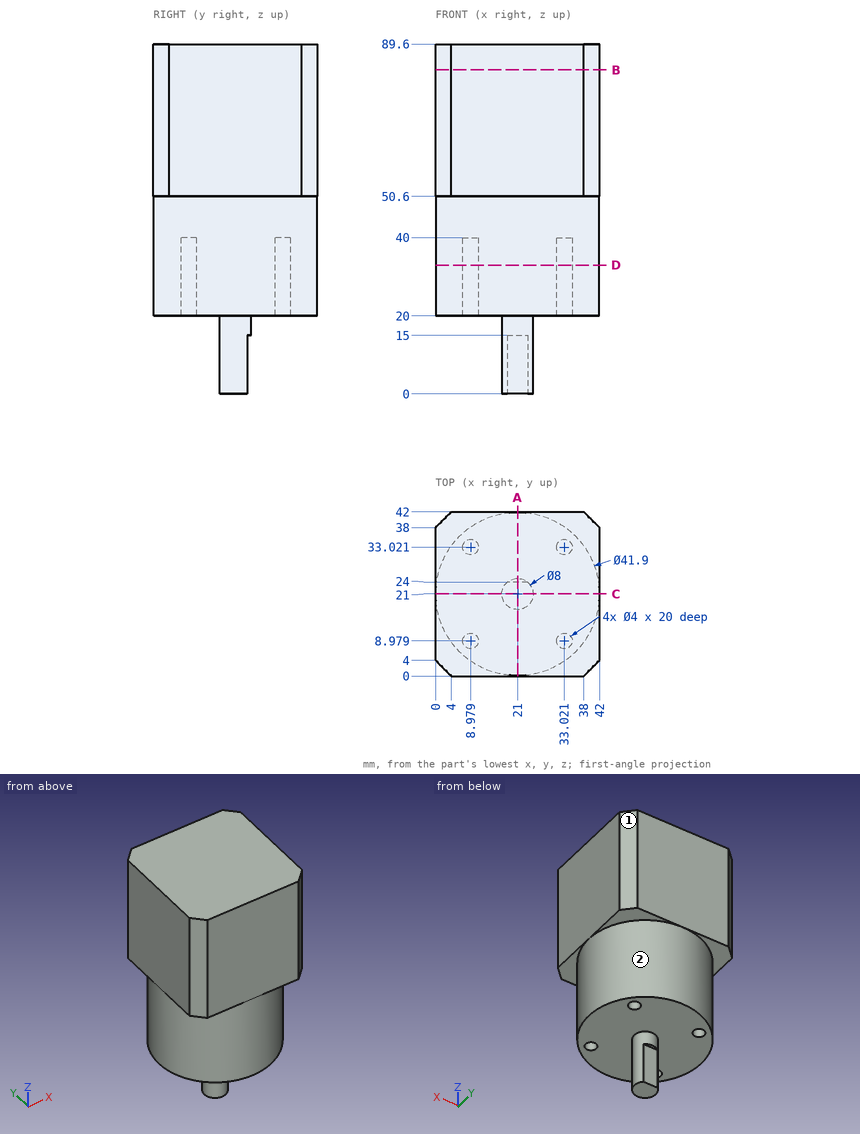
The drawing under review shows one solid part. Ordinate dimensions are in mm from its lowest x, y, z. A direction names the side the tool comes from. Give positions to 0.01 mm unless a question says otherwise; leave off trailing zeros. Order: outer loops, then holes, each group sorted by start corner. A loop starts at its lowest first (then second) coordinate and runs counter-clockwise, first axis right, second up. Notation, with made-up numbers: (38, 35.5) -> (61, 35.5) arc R33 cw to (61, 74.5) -> close; hole circle Ø11 at (-17, -27). An arc over 180 degrees is marked (long way). Write item = value, one per line.
1) We need section B-B, the plane z = 83. Give the boundary of the cut face in (x, y).
Findings:
outline = (0, 4) -> (4, 0) -> (38, 0) -> (42, 4) -> (42, 38) -> (38, 42) -> (4, 42) -> (0, 38) -> close
2) We need section D-D, the plane z = 33. Give the boundary of the cut face in (x, y).
Findings:
outline = circle Ø41.9 at (21, 21); hole circle Ø4 at (8.98, 8.98); hole circle Ø4 at (8.98, 33.02); hole circle Ø4 at (33.02, 8.98); hole circle Ø4 at (33.02, 33.02)
3) To check wall thickness, follow L1, parallel to Y at x = 8.5, z = 31.5; L2, parallel to X at y = 8, z = 25 (1 decimal); L3, parallel to Z at x = 2, y = 26.5. State the ranges of each line that lie inside material, in increasing order. Write a range as from..to.
Findings:
L1 = 4.19..7.04, 10.92..31.08, 34.96..37.81
L2 = 4.6..7.2, 10.7..31.3, 34.8..37.4
L3 = 20..89.6
4) We need section A-A, the plane x = 21. Give the boundary of the cut face in (y, z), and give its area (3 significant figures).
Findings:
outline = (0, 50.6) -> (0.05, 50.6) -> (0.05, 20) -> (17, 20) -> (17, 0) -> (24, 0) -> (24, 15) -> (25, 15) -> (25, 20) -> (41.95, 20) -> (41.95, 50.6) -> (42, 50.6) -> (42, 89.6) -> (0, 89.6) -> close
area = 3,070 mm^2
5) Insertion check: pin 1 (4.5 mm diameter, centred on x = 32, y = 8.5, fed in from -Z); pin 2 (4 mm diameter, centred on x = 20, z = 4, fed in from +Y); pin 3 (1 mm diameter, centred on y = 16.5, z = 25, fed in from +X). Each pin has a flat end and moves straight along its axis. Give the tip position at first contact, or say it passes through.
Findings:
pin_1 = 20
pin_2 = 24
pin_3 = 41.56
6) For the marked faces 1 and 2, list the 3-axis set-ups (+Z, -Z, +X, -X, +Y, -Y) from which the entire face can be reached by the end or side of a thin tool; tool diameter is ignored.
Findings:
face_1 = +Z, -Z, +X, +Y
face_2 = -Z
7) We need section C-C, the plane y = 21. Give the boundary of the cut face in (x, z).
Findings:
outline = (0, 50.6) -> (0.05, 50.6) -> (0.05, 20) -> (17, 20) -> (17, 0) -> (25, 0) -> (25, 20) -> (41.95, 20) -> (41.95, 50.6) -> (42, 50.6) -> (42, 89.6) -> (0, 89.6) -> close
